```python
from build123d import *
from OCP.BRepFilletAPI import BRepFilletAPI_MakeChamfer

# Parameters (mm, degrees)
EXTRUDE_1_DEPTH       = 15
SKETCH_2_W            = 12
SKETCH_2_H            = 31.380738368
CUT_EXTRUDE_2_DEPTH   = 78.211371281
CHAMFER_1_SIZE        = 3
CHAMFER_1_SIZE2       = 3.575260778
SKETCH_4_R            = 2.5
CUT_EXTRUDE_3_DEPTH   = 86.823049672
SKETCH_8_R            = 1.5
CUT_EXTRUDE_3_2_DEPTH = 100.757006451
CUT_EXTRUDE_4_DEPTH   = 100.757006451
SKETCH_11_W           = 1.5
SKETCH_11_H           = 83.943010544
SKETCH_11_H_2         = 90.462059893
CUT_EXTRUDE_6_DEPTH   = 1.5
FILLET_7_R            = 4


with BuildPart() as part:
    # Эскиз1 → Вытянуть1 (new body)
    with BuildSketch(Plane(origin=(0, 0, 0), x_dir=(1, 0, 0), z_dir=(0, 1, 0))):
        Polygon((-39.391292545, -35), (47.5, -35), (47.5, 41.994456138), (41.467636093, 41.994456138), (41.467636093, 58.994456138), (34.467636093, 58.994456138), (34.467636093, 41.994456138), (19.467636417, 41.994456138), (19.467636417, 58.994456138), (12.467636275, 58.994456138), (12.467636275, 41.994456138), (-2.532363543, 41.994456138), (-2.532363543, 58.994456138), (-9.532363543, 58.994456138), (-9.532363543, 41.994456138), (-24.532363361, 41.994456138), (-24.532363361, 58.994456138), (-31.532363503, 58.994456138), (-31.532363503, 41.994456138), (-39.391292545, 41.994456138), align=None)
    extrude(amount=EXTRUDE_1_DEPTH)

    # Эскиз2 → Вытянуть2 (cut, through all)
    with BuildSketch(Plane(origin=(0, 15, 0), x_dir=(1, 0, 0), z_dir=(0, 1, 0))):
        with Locations((0, -35)):
            Rectangle(SKETCH_2_W, SKETCH_2_H)
        Polygon((-40.282255649, -10.968321), (-13, -19.309630816), (-13, -35), (-40.282255649, -35), align=None)
        Polygon((49.575798338, -35), (13, -35), (13, -19.309630816), (49.575798338, -9.764075531), align=None)
    extrude(amount=-CUT_EXTRUDE_2_DEPTH, mode=Mode.SUBTRACT)

    # Фаска1: one chamfer whose edges measure the first distance from different faces: ONE call of the kernel's chamfer builder (chamfer() names one face for all edges)
    chamfer_1_edges_1 = [part.edges().sort_by_distance(p)[0] for p in [
        (9.5, 0, 35),
        (-9.5, 0, 35),
    ]]
    chamfer_1_side_1 = [part.faces().sort_by_distance(p)[0] for p in [
        (3.754326558, 0, -14.37188085),
    ]]
    chamfer_1_edges_2 = [part.edges().sort_by_distance(p)[0] for p in [
        (9.5, 15, 35),
    ]]
    chamfer_1_side_2 = [part.faces().sort_by_distance(p)[0] for p in [
        (9.5, 7.5, 35),
    ]]
    chamfer_1_edges_3 = [part.edges().sort_by_distance(p)[0] for p in [
        (-9.5, 15, 35),
    ]]
    chamfer_1_side_3 = [part.faces().sort_by_distance(p)[0] for p in [
        (-9.5, 7.5, 35),
    ]]
    chamfer_1 = BRepFilletAPI_MakeChamfer(part.part.solid().wrapped)
    for e in chamfer_1_edges_1:
        chamfer_1.Add(CHAMFER_1_SIZE, CHAMFER_1_SIZE2, e.wrapped, chamfer_1_side_1[0].wrapped)  # the first distance lies on this face
    for e in chamfer_1_edges_2:
        chamfer_1.Add(CHAMFER_1_SIZE, CHAMFER_1_SIZE2, e.wrapped, chamfer_1_side_2[0].wrapped)  # the first distance lies on this face
    for e in chamfer_1_edges_3:
        chamfer_1.Add(CHAMFER_1_SIZE, CHAMFER_1_SIZE2, e.wrapped, chamfer_1_side_3[0].wrapped)  # the first distance lies on this face
    add(Compound.cast(chamfer_1.Shape()), mode=Mode.REPLACE)

    # Эскиз4 → Cut-Extrude 3 (cut, through all)
    with BuildSketch(Plane.ZY.offset(13)):
        with Locations((27.080154825, 7.787630389)):
            Circle(SKETCH_4_R)
    extrude(amount=-CUT_EXTRUDE_3_DEPTH, mode=Mode.SUBTRACT)

    # Эскиз8 → Cut-Extrude 3 2 (cut, through all)
    with BuildSketch(Plane.ZY.offset(31.532363503)):
        with Locations((-52.695808176, 5.099933888)):
            Circle(SKETCH_8_R)
    extrude(amount=-CUT_EXTRUDE_3_2_DEPTH, mode=Mode.SUBTRACT)

    # Эскиз9 → Вырез-Вытянуть4 (cut, through all)
    with BuildSketch(Plane.ZY.offset(31.532363503)):
        Polygon((-47.921961808, 15), (-55.921789721, 7.000172087), (-55.921789721, 3.000172087), (-52.921609925, -7.709e-06), (-58.994456138, -7.709e-06), (-58.994456138, 15), align=None)
    extrude(amount=-CUT_EXTRUDE_4_DEPTH, mode=Mode.SUBTRACT)

    # Эскиз11 → Вырез-Вытянуть6 (cut)
    with BuildSketch(Plane.XZ):
        with Locations((37.967637049, -4.77082371)):
            Rectangle(SKETCH_11_W, SKETCH_11_H)
        with Locations((-6.032362804, -4.77082371)):
            Rectangle(SKETCH_11_W, SKETCH_11_H)
        with Locations((15.967637122, -1.511299036)):
            Rectangle(SKETCH_11_W, SKETCH_11_H_2)
        with Locations((-28.032362511, -1.511299036)):
            Rectangle(SKETCH_11_W, SKETCH_11_H_2)
    extrude(amount=-CUT_EXTRUDE_6_DEPTH, mode=Mode.SUBTRACT)

    # Скругление7
    fillet_7_edges = [part.edges().sort_by_distance(p)[0] for p in [
        (41.467636093, 7.5, -41.994456138),
        (34.467636093, 7.5, -41.994456138),
        (19.467636417, 7.5, -41.994456138),
        (12.467636275, 7.5, -41.994456138),
        (-2.532363543, 7.5, -41.994456138),
        (-9.532363543, 7.5, -41.994456138),
        (-24.532363361, 7.5, -41.994456138),
        (-31.532363503, 7.5, -41.994456138),
    ]]
    fillet(fillet_7_edges, radius=FILLET_7_R)


solid = part.part
```
Can you work these out from the model? Positions are in its coordinate system, mm. A direction names the side the tool comes from. Round coordinates to 2 decimals unless told otherwise and drop trailing zeros. Loops run counter-clockwise (first coordinate to the right, second up) from the corner with the lowest first, then second, coordinate; pieces in that order, holes last. Notation, with made-up numbers: M -29,68 L -23,68 A10 cw -23,86 Z; hole C -37.5,-36 d8. An arc over 180 degrees is marked long. Answer in a Markdown table with one row per item.
1. Please list where these lines run through material, in increasing order: line 1 (X direction, y = 11.5, z = 25.5); line 2 (X direction, y = 4.25, z = -43); line 3 (Z direction, x = 21, y = 4). Write a range as from..to.
Established:
| item | result |
|---|---|
| line 1 | -13..-6, 6..13 |
| line 2 | -32.88..-23.18, -10.88..-1.18, 11.12..20.82, 33.12..42.82 |
| line 3 | -42.85..17.22 |
2. If we section it at B-B, the plane z = 23.5: Please give me the cut outline in (x, y), plus the area to 3 significant figures.
Established:
| item | result |
|---|---|
| outline | M -13,0 L -6.78,0 L -6.78,1.5 L -6,1.5 L -6,15 L -13,15 Z; M 6,0 L 13,0 L 13,15 L 6,15 Z |
| area | 209 mm² |
3. If we section it at D-D, the plane x = 21.5: Please give me the cut outline in (y, z).
Established:
| item | result |
|---|---|
| outline | M 0,-42.51 L 15,-42.51 L 15,17.09 L 0,17.09 Z |
4. If we section it at A-A, the plane z = -44.5: Give the number of separate pieces and of enclosed holes in the cut face, plus the area to 3 significant figures.
Established:
| item | result |
|---|---|
| separate pieces | 4 |
| enclosed holes | 0 |
| area | 446 mm² |
5. On a 3-axis mill with a long thin cutter (end or side, diameter ignored), from which of +Z, -Z, +X, -X, +Y, -Y can I reach the whole of each face in a straight line? I mean faces 1 (the face through (-13, 6, 25)), 2 (the face through (-1.392, 7.605, -43.197)), 3 (the face through (37.919, 11.056, -51.866)), 4 (the face through (13, 5.9, 29)). Say none if no direction works.
Established:
| item | result |
|---|---|
| face 1 | +Z, -X, +Y, -Y |
| face 2 | -Z, +Y, -Y |
| face 3 | -Z, +X, -X, +Y |
| face 4 | +Z, +X, +Y, -Y |
6. I'm going to push flat-ended pins straight in: pin 1 Ø1.6 at (x, y) = (15.5, 0.5) entering from +Z; pin 2 Ø5 at (y, z) = (9, -51.5) entering from -X; pin 3 Ø7.5 at (y, z) = (4.5, 28.5) entering from +X. Where does each tip first touch, or does it pass through?
Established:
| item | result |
|---|---|
| pin 1 | z = 18.87 |
| pin 2 | x = -31.53 |
| pin 3 | x = 13 |
7. Thinking about a two-plate mould opening in Z: for faces 5 (the face through (9, 8, 35)), 6 (the face through (-9.532, 6, -50)), 7 (the face through (-9.55, 6.83, 29.39)), which applies, pulls with the +Z half, pulls with the -Z half, needs draft (parallel to the pull), parting line crosses it, or undercut?
Established:
| item | result |
|---|---|
| face 5 | pulls with the +Z half |
| face 6 | needs draft |
| face 7 | undercut |
